Source: CAD feature listing. Evaluate the final solid. Frame: model axes, mm. A direction names the side the tool comes from. Give positions to 0.01 mm unless a question says otherwise; leave off trailing zeros. Order: outer loops, then holes, each group sorted by start corner. A loop starts at its lowest first (then second) coordinate and runs counter-clockwise, first axis right, second up.
from build123d import *

# Parameters (mm, degrees)
SKETCH1_W               = 76.2
SKETCH1_H               = 25.4
SKETCH1_W_2             = 69.85
SKETCH1_H_2             = 19.05
BOSS_EXTRUDE1_DEPTH     = 254
SKETCH3_R               = 3.3782
CUT_EXTRUDE1_DEPTH      = 26.4
SKETCH4_R               = 3.3782
CUT_EXTRUDE2_DEPTH      = 1
CUT_EXTRUDE2_DEPTH_BACK = 77.2


with BuildPart() as part:
    # Sketch1 → Boss-Extrude1 (new body)
    with BuildSketch(Plane(origin=(0, 0, 0), x_dir=(1, 0, 0), z_dir=(0, 1, 0))):
        with Locations((38.1, 12.7)):
            Rectangle(SKETCH1_W, SKETCH1_H)
        with Locations((38.1, 12.7)):
            Rectangle(SKETCH1_W_2, SKETCH1_H_2, mode=Mode.SUBTRACT)
    extrude(amount=BOSS_EXTRUDE1_DEPTH)

    # Sketch3 → Cut-Extrude1 (cut, through all)
    with BuildSketch(Plane.XY):
        with Locations((56.897712706, 53.783695383)):
            Circle(SKETCH3_R)
        with Locations((18.636431119, 102.638247629)):
            Circle(SKETCH3_R)
        with Locations((33.330604718, 127.14563197)):
            Circle(SKETCH3_R)
    extrude(amount=-CUT_EXTRUDE1_DEPTH, mode=Mode.SUBTRACT)

    # Sketch4 → Cut-Extrude2 (cut, two sides)
    with BuildSketch(Plane.ZY) as cut_extrude2_sk:
        with Locations((-12.7, 237.7313)):
            Circle(SKETCH4_R)
    extrude(amount=CUT_EXTRUDE2_DEPTH, mode=Mode.SUBTRACT)
    extrude(cut_extrude2_sk.sketch, amount=-CUT_EXTRUDE2_DEPTH_BACK, mode=Mode.SUBTRACT)


solid = part.part
1) First-contact query: pin 1 Ø8 at (x, y) = (18.64, 102.64) entering from +Z. Flat tip, straight axial feed; report the tip coordinate or a pass-through.
Checks:
pin 1: stops at z = 0
2) Ray query, L1, parallel to Z at x = 27, y = 233 (3 decimals); L2, parallel to X at y = 123, z = -6.75 (3 decimals); L3, parallel to Y at x = 57.5, z = -23. Return the intervals inside material, ascending.
Checks:
L1: z = -25.4 to -22.225, -3.175 to 0
L2: x = 0 to 3.175, 73.025 to 76.2
L3: y = 0 to 50.46, 57.11 to 254
3) Section query C-C on y = 77.5. Output: boundary loops of the cut face in (x, z) (3 decimals), and give its area (3 significant figures).
Checks:
outline: (0, -25.4) - (76.2, -25.4) - (76.2, 0) - (0, 0) - close; hole (3.175, -22.225) - (73.025, -22.225) - (73.025, -3.175) - (3.175, -3.175) - close
area: 605 mm2
4) Section query A-A on z = -12.7. Output: boundary loops of the cut face in (x, y) (1 decimal), and give its area (3 significant figures).
Checks:
outline: (0, 0) - (3.2, 0) - (3.2, 234.4) - (0, 234.4) - close; (0, 241.1) - (3.2, 241.1) - (3.2, 254) - (0, 254) - close; (73, 0) - (76.2, 0) - (76.2, 234.4) - (73, 234.4) - close; (73, 241.1) - (76.2, 241.1) - (76.2, 254) - (73, 254) - close
area: 1,570 mm2
5) Reachability of faces 1 (the face through (38, 125, -22.225)), 2 (the face through (58.714, 56.632, -1.565)) from +Z, -Z, +X, -X, +Y, -Y: full face, straight path, thin tool, end or side. Return the list, or none.
Checks:
face 1: +Y, -Y
face 2: +Z, -Z
6) Section query B-B on x = 70. Output: boundary loops of the cut face in (y, z) (3 decimals), and give its area (3 significant figures).
Checks:
outline: (0, -25.4) - (254, -25.4) - (254, -22.225) - (0, -22.225) - close; (0, -3.175) - (254, -3.175) - (254, 0) - (0, 0) - close
area: 1,610 mm2
7) Pull-direction query (Z, two-part tool) for faces 3 (the face through (35.15, 129.99, -1.57)), 4 (the face through (1.57, 241.08, -13.14)), 5 (the face through (38, 125, 0)); classes: +Z half, -Z half, draft (parallel to the pull), parting line (faces both ways), or undercut.
Checks:
face 3: draft
face 4: undercut
face 5: +Z half
8) Section query D-D on x = 56. Output: boundary loops of the cut face in (y, z) (3 decimals), and give its area (3 significant figures).
Checks:
outline: (0, -25.4) - (50.527, -25.4) - (50.527, -22.225) - (0, -22.225) - close; (0, -3.175) - (50.527, -3.175) - (50.527, 0) - (0, 0) - close; (57.04, -25.4) - (254, -25.4) - (254, -22.225) - (57.04, -22.225) - close; (57.04, -3.175) - (254, -3.175) - (254, 0) - (57.04, 0) - close
area: 1,570 mm2
